Answer from the drawing. Dimensions are ordinates in mm from the lowest x, y and z of the part. A direction names the side the tool comes from. Round coordinates to 2 decimals unless told otherwise and drop trailing zeros. Write each loop counter-clockwise with the first axis right and the second up, starting at its lowest first coordinate (ties: lowest second). Pieces come first, ordered by that corner, then holes. Notation, with made-up numbers: (-32.75, -0.75) - (18.25, -0.75) arc R20 cw to (18.25, 4.25) - close; hole circle Ø9 at (41.25, 46). An arc over 180 degrees is marked (long way). One line per item, written item: value. Start each with the question number.
(1) For the marked faces 1, 2 and 3, determine the directions among +Z, -Z, +X, -X, +Y, -Y from which every point of the face is accessible in a straight line to the end or side of a thin tool.
(2) A cutting plane is placed at D-D, the plane z = 45. Determine the outline of the cut face in (x, y), plus the area to 3 significant figures.
(3) A cutting plane is placed at C-C, the plane x = 28.5. Determine the outline of the cut face in (y, z).
(4) A cutting plane is placed at B-B, the plane y = 37. Determine the outline of the cut face in (x, z), plus the area to 3 significant figures.
(5) Flat-ended cylindrical pins translate along their axes: pin 1 Ø12 at (x, z) = (66, 28) entering from +Y; pin 2 Ø10 at (x, y) = (90.5, 20) entering from +Z; pin 3 Ø5 at (y, z) = (41.5, 16) entering from -X. Find the tip coordinate at first contact, or state that the pin passes through.
(6) Find the intervals of material crossed by L1, parallel to X at y = 33, z = 11; L2, parallel to X at y = 10, z = 28; L3, parallel to Z at x = 70, y = 28, in increasing order.
(7) A cutting plane is placed at A-A, the plane z = 29. Determine the outline of the cut face in (x, y).
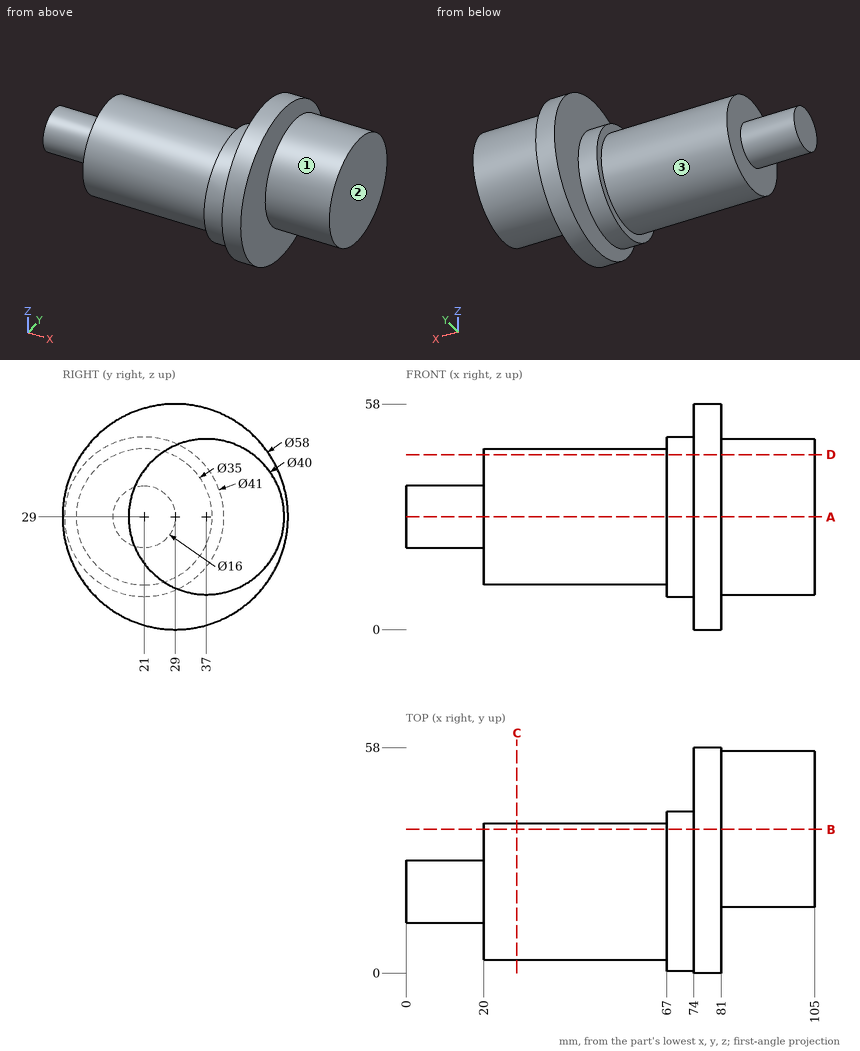
Here are the results:
1. face 1: +X
1. face 2: +Z, -Z, +X, +Y, -Y
1. face 3: -X
2. outline: (20, 13.91) - (67, 13.91) - (67, 8.18) - (74, 8.18) - (74, 4.81) - (81, 4.81) - (81, 25) - (105, 25) - (105, 49) - (81, 49) - (81, 53.19) - (74, 53.19) - (74, 33.82) - (67, 33.82) - (67, 28.09) - (20, 28.09) - close
2. area: 1,760 mm²
3. outline: circle Ø35 at (21, 29)
4. outline: (20, 21.91) - (67, 21.91) - (67, 16.18) - (74, 16.18) - (74, 1.13) - (81, 1.13) - (81, 9) - (105, 9) - (105, 49) - (81, 49) - (81, 56.87) - (74, 56.87) - (74, 41.82) - (67, 41.82) - (67, 36.09) - (20, 36.09) - close
4. area: 2,200 mm²
5. pin 1: y = 41.5
5. pin 2: z = 45
5. pin 3: x = 74
6. L1: 74 to 105
6. L2: 20 to 81
6. L3: 9.73 to 48.27
7. outline: (0, 13) - (20, 13) - (20, 3.5) - (67, 3.5) - (67, 0.5) - (74, 0.5) - (74, 0) - (81, 0) - (81, 17) - (105, 17) - (105, 57) - (81, 57) - (81, 58) - (74, 58) - (74, 41.5) - (67, 41.5) - (67, 38.5) - (20, 38.5) - (20, 29) - (0, 29) - close
